Read the model definition and answer for the solid it produces. Units are mm, in the model's axes. Give positions to 0.01 mm unless a question says otherwise; leave off trailing zeros. Use a Markdown table: item, result. Add a question column.
1. Flat-ended cylindrical pins translate along their axes: P1, Ø2.5, axis at x = 436.5, z = 2, coming from the +Y side; P2, Ø2.5, axis at y = 162.5, z = 2.5, coming from the +X side. Find the tip coordinate at first contact, or state that the pin passes through.
2. Consider L1, parallel to Y at x = 80, z = 3; L2, parallel to X at y = 160.5, z = 3.8; L3, parallel to Y at x = 70, z = 3.35. Determine where each line is inside the solid, lowest interval first.
3. A cutting plane is placed at A-A on z = 3.2. State how many separate pieces and enclosed holes the cut face has, and give its area (3 significant figures).
```python
from build123d import *

# Parameters (mm, degrees)
F0_R     = 2.25
F0_W     = 6
F0_H     = 2
F0_R_2   = 3
F1_DEPTH = 5


with BuildPart() as f1:
    # F0 (on Top) → F1 (new body)
    with BuildSketch(Plane.XY):
        with BuildLine():
            ThreePointArc((-150, -7.5), (-149.414214, -8.914214), (-148, -9.5))
            Line((-148, -9.5), (448, -9.5))
            ThreePointArc((448, -9.5), (449.414214, -8.914214), (450, -7.5))
            Line((450, -7.5), (450, 150.5))
            Line((450, 150.5), (429.5, 150.5))
            Line((429.5, 150.5), (429.5, 170.5))
            Line((429.5, 170.5), (210, 170.5))
            Line((210, 170.5), (210, 150.5))
            Line((210, 150.5), (90, 150.5))
            Line((90, 150.5), (90, 170.5))
            Line((90, 170.5), (-129.5, 170.5))
            Line((-129.5, 170.5), (-129.5, 150.5))
            Line((-129.5, 150.5), (-150, 150.5))
            Line((-150, 150.5), (-150, -7.5))
        make_face()
        with Locations((-140, 0.5)):
            Circle(F0_R, mode=Mode.SUBTRACT)
        with Locations((-60, -4)):
            Rectangle(F0_W, F0_H, mode=Mode.SUBTRACT)
        with Locations((-70, 0)):
            Circle(F0_R_2, mode=Mode.SUBTRACT)
        with Locations((-60, 4)):
            Rectangle(F0_W, F0_H, mode=Mode.SUBTRACT)
        with Locations((70, 0)):
            Circle(F0_R_2, mode=Mode.SUBTRACT)
        with Locations((80, -4)):
            Rectangle(F0_W, F0_H, mode=Mode.SUBTRACT)
        with Locations((80, 4)):
            Rectangle(F0_W, F0_H, mode=Mode.SUBTRACT)
        with Locations((220, -4)):
            Rectangle(F0_W, F0_H, mode=Mode.SUBTRACT)
        with Locations((220, 4)):
            Rectangle(F0_W, F0_H, mode=Mode.SUBTRACT)
        with Locations((230, 0)):
            Circle(F0_R_2, mode=Mode.SUBTRACT)
        with Locations((360, -4)):
            Rectangle(F0_W, F0_H, mode=Mode.SUBTRACT)
        with Locations((370, 0)):
            Circle(F0_R_2, mode=Mode.SUBTRACT)
        with Locations((360, 4)):
            Rectangle(F0_W, F0_H, mode=Mode.SUBTRACT)
        with Locations((440, 0.5)):
            Circle(F0_R, mode=Mode.SUBTRACT)
        with Locations((80, 160.5)):
            Circle(F0_R, mode=Mode.SUBTRACT)
    extrude(amount=F1_DEPTH)


solid = f1.part
```
Output values:
| question | item | result |
|---|---|---|
| 1 | P1 | y = 150.5 |
| 1 | P2 | x = 429.5 |
| 2 | L1 | -9.5 to -5, -3 to 3, 5 to 158.25, 162.75 to 170.5 |
| 2 | L2 | -129.5 to 77.75, 82.25 to 90, 210 to 429.5 |
| 2 | L3 | -9.5 to -3, 3 to 170.5 |
| 3 | separate pieces | 1 |
| 3 | enclosed holes | 15 |
| 3 | area | 105,000 mm² |
